Print and shaded views of the part. All mm, measured from the part's lowest x, y and z. Give positions to 0.01 mm unless a question says otherwise; leave off trailing zeros. Loops run counter-clockwise (first coordinate to the right, second up) from the corner with the lowest first, then second, coordinate; pieces in that order, holes last.
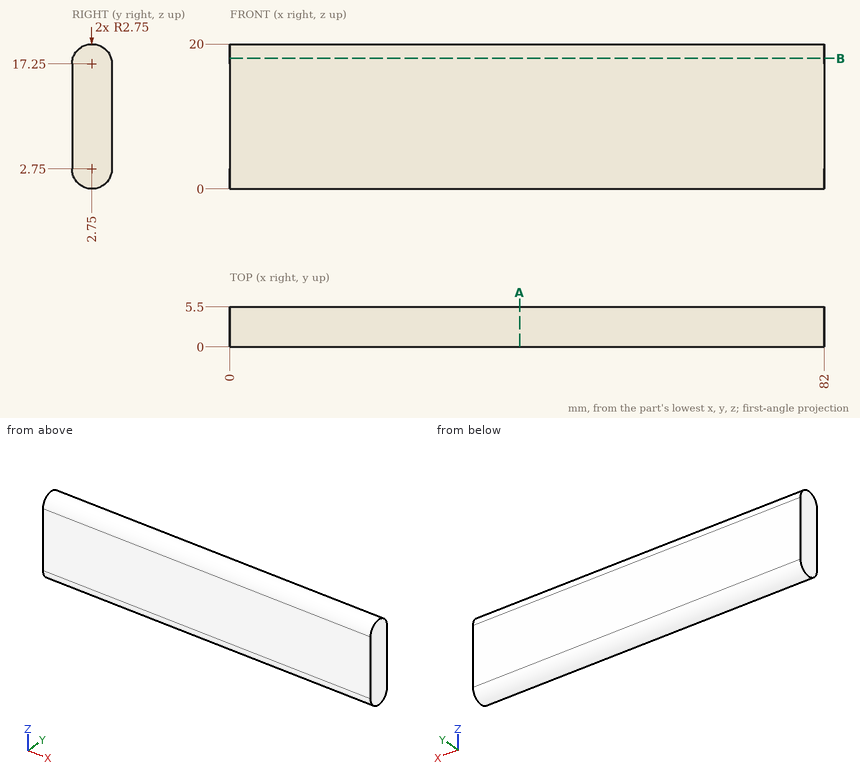
1. Saw through at A-A, the plane x = 40. List the corners of the cut face in (y, z).
Responses:
outline: (0, 2.75) arc R2.75 ccw to (5.5, 2.75) - (5.5, 17.25) arc R2.75 ccw to (0, 17.25) - close
2. Saw through at B-B, the plane z = 18. List the corners of the cut face in (x, y), and give its area (3 significant figures).
Responses:
outline: (0, 0.1) - (82, 0.1) - (82, 5.4) - (0, 5.4) - close
area: 434 mm2
3. Probe line 1 along Z through (x, y) = (60, 3.05); line 2 along Y through (x, z) = (70, 17.5); line 3 along Z through (x, y) = (68, 1.85). List the from-to ranges inside material, lowest first.
Responses:
line 1: z = 0.02 to 19.98
line 2: y = 0.01 to 5.49
line 3: z = 0.15 to 19.85
